```python
from build123d import *

# Parameters (mm, degrees)
Y_KSEKLIK_EKSTR_ZYON1_DEPTH = 38
IZIM2_W                     = 31
IZIM2_H                     = 30
KES_EKSTR_ZYON1_DEPTH       = 33.5
KES_EKSTR_ZYON2_DEPTH       = 38
KES_EKSTR_ZYON3_DEPTH       = 38
RADYUS2_R                   = 2


with BuildPart() as part:
    # Çizim1 → Yükseklik-Ekstrüzyon1 (new body)
    with BuildSketch(Plane(origin=(0, 0, 0), x_dir=(0, 0, -1), z_dir=(1, 0, 0))):
        Polygon((0, 0), (0, 37), (3.5, 37), (3.5, 33.5), (33.5, 3.5), (37, 3.5), (37, 0), align=None)
    extrude(amount=Y_KSEKLIK_EKSTR_ZYON1_DEPTH)

    # Çizim2 → Kes-Ekstrüzyon1 (cut)
    with BuildSketch(Plane(origin=(0, 0, -37), x_dir=(-1, 0, 0), z_dir=(0, 0, -1))):
        with Locations((-19, 18.5)):
            Rectangle(IZIM2_W, IZIM2_H)
    extrude(amount=-KES_EKSTR_ZYON1_DEPTH, mode=Mode.SUBTRACT)

    # Çizim3 → Kes-Ekstrüzyon2 (cut)
    with BuildSketch(Plane(origin=(0, 0, -3.5), x_dir=(-1, 0, 0), z_dir=(0, 0, -1))):
        with BuildLine():
            Line((-14.6, 22.5), (-14.6, 14.5))
            ThreePointArc((-14.6, 14.5), (-19, 10.1), (-23.4, 14.5))
            Line((-23.4, 14.5), (-23.4, 22.5))
            ThreePointArc((-23.4, 22.5), (-19, 26.9), (-14.6, 22.5))
        make_face()
    extrude(amount=-KES_EKSTR_ZYON2_DEPTH, mode=Mode.SUBTRACT)

    # Çizim4 → Kes-Ekstrüzyon3 (cut)
    with BuildSketch(Plane(origin=(0, 3.5, 0), x_dir=(1, 0, 0), z_dir=(0, 1, 0))):
        with BuildLine():
            Line((23.4, 22.5), (23.4, 14.5))
            ThreePointArc((23.4, 14.5), (19, 10.1), (14.6, 14.5))
            Line((14.6, 14.5), (14.6, 22.5))
            ThreePointArc((14.6, 22.5), (19, 26.9), (23.4, 22.5))
        make_face()
    extrude(amount=-KES_EKSTR_ZYON3_DEPTH, mode=Mode.SUBTRACT)

    # Radyus2
    radyus2_edges = [part.edges().sort_by_distance(p)[0] for p in [
        (38, 37, -1.75),
        (38, 1.75, -37),
        (0, 37, -1.75),
        (0, 1.75, -37),
    ]]
    fillet(radyus2_edges, radius=RADYUS2_R)


solid = part.part
```
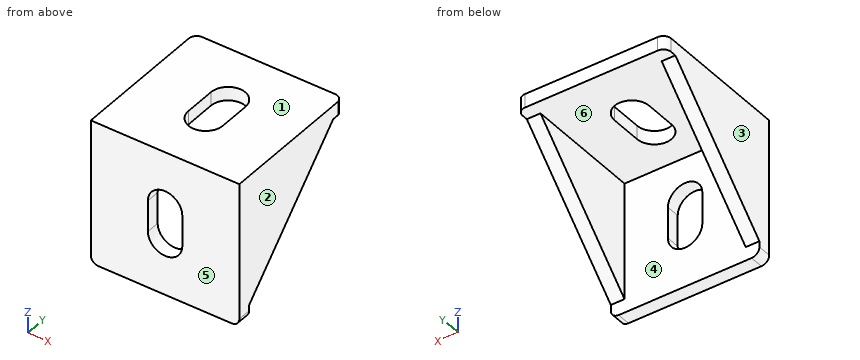
Geometry: final body of the model. Coordinates: model frame, mm. Face numbers are marked on the shaded views. A direction names the side the tool comes from. Coordinates: 2 decimals unless noted, no trailing zeros. Write each loop counter-clockwise with the first axis right and the second up, starting at its lowest first coordinate (ties: lowest second). Pieces come first, ordered by that corner, then holes. Notation, with made-up numbers: M 29.25,33.5 L 51.25,33.5 A27 ccw 51.25,60.5 Z; hole C 24.5,31.5 d6. An arc over 180 degrees is marked long. Use CSV: the item, a comma, the result in double quotes. Start each with the question number.
1. First-contact query: P1, Ø8, axis at x = 13, y = 19, coming from the -Z side; P2, Ø10, axis at x = 25.5, z = -27, coming from the +Y side; P3, Ø9, axis at y = 25.5, z = -18.5, coming from the -X side. Flat tips, straight axial feed; report the tip coordinate or a pass-through.
2. Cut plane D-D on y = 9.5. Return the cut outline in (x, z), plus the area to 3 significant figures.
3. Ray query, probe 1 along X at (y, z) = (5, -17); probe 2 along Y at (x, z) = (5, -6); probe 3 along Z at (x, y) = (5.5, 14.5). Return the intervals inside material, ascending.
4. Mould query, pull axis X, two halves, no side actions, for the marked faces 1, 2, 3 and 4. Classes: pulls with the +X half, pulls with the -X half, needs draft (parallel to the pull), parting line crosses it, or undercut.
5. Reachability of the marked faces 5 and 6 from +Z, -Z, +X, -X, +Y, -Y: full face, straight path, thin tool, end or side. Return the list, or none.
6. Cut plane C-C on x = 19. Return the cut outline in (y, z), plus the area to 3 significant figures.
7. Cut plane A-A on y = 18.5. Return the cut outline in (x, z).
8. Cut plane B-B on z = -17. Return the cut outline in (x, y).
Entries:
1,P1,"z = -3.5"
1,P2,"y = 3.5"
1,P3,"through"
2,outline,"M 0,-27.5 L 3.5,-27.5 L 3.5,-3.5 L 34.5,-3.5 L 34.5,-27.5 L 38,-27.5 L 38,0 L 0,0 Z"
2,area,"301 mm²"
3,probe 1,"0 to 3.5, 34.5 to 38"
3,probe 2,"0 to 3.5"
3,probe 3,"-3.5 to 0"
4,face 1,"needs draft"
4,face 2,"pulls with the +X half"
4,face 3,"pulls with the -X half"
4,face 4,"undercut"
5,face 5,"+Z, -Z, +X, -X, -Y"
5,face 6,"-Z, +Y"
6,outline,"M 0,-37 L 3.5,-37 L 3.5,-26.9 L 0,-26.9 Z; M 0,-10.1 L 3.5,-10.1 L 3.5,-3.5 L 10.1,-3.5 L 10.1,0 L 0,0 Z; M 26.9,-3.5 L 37,-3.5 L 37,0 L 26.9,0 Z"
6,area,"129 mm²"
7,outline,"M 0,-18.5 L 3.5,-18.5 L 3.5,-3.5 L 14.6,-3.5 L 14.6,0 L 0,0 Z; M 23.4,-3.5 L 34.5,-3.5 L 34.5,-18.5 L 38,-18.5 L 38,0 L 23.4,0 Z"
8,outline,"M 0,0 L 14.6,0 L 14.6,3.5 L 3.5,3.5 L 3.5,20 L 0,20 Z; M 23.4,0 L 38,0 L 38,20 L 34.5,20 L 34.5,3.5 L 23.4,3.5 Z"
